Can you work these out from the model? Positions are in its coordinate system, mm. Face numbers are marked on the shaded views. A direction names the side the tool comes from. Give positions to 0.01 mm unless a question says otherwise; leave off trailing zeros. Write each loop counter-clockwise with the first axis right and the second up, starting at its lowest first coordinate (ties: lowest second). Pieces come first, ordered by that corner, then holes. Notation, with made-up numbers: M 13.5,62.25 L 25.5,62.25 A18 ccw 25.5,74.25 Z; hole C 38,-21 d7. An arc over 180 degrees is marked long. Answer as CSV lines item,"result". Start each with the question number.
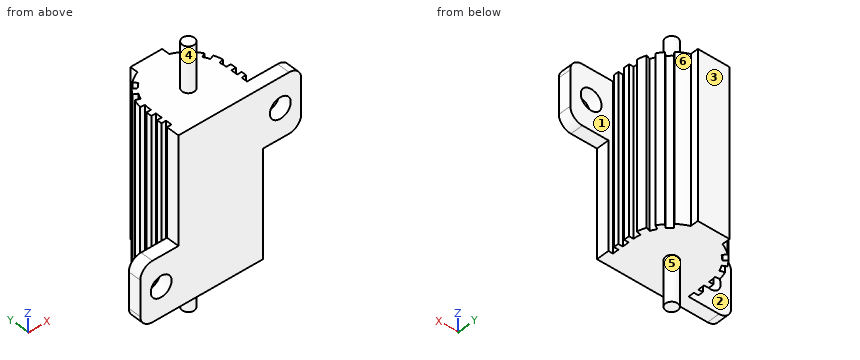
```python
from build123d import *

# Parameters (mm, degrees)
EXTRUDE1_DEPTH     = 14
SKETCH4_W          = 6.4
SKETCH4_H          = 10
EXTRUDE8_DEPTH     = 2.159
FILLET1_R          = 2.032
CUT_EXTRUDE1_START = -28
SKETCH3_W          = 0.762
SKETCH3_H          = 1.095986398
SKETCH3_H_2        = 1.017694432
CUT_EXTRUDE1_DEPTH = 28
SKETCH5_R          = 1.75
CUT_EXTRUDE2_DEPTH = 3.159
SKETCH6_R          = 1.02616
EXTRUDE9_DEPTH     = 7.62


with BuildPart() as part:
    # Sketch2 → Extrude1 (new body, symmetric)
    with BuildSketch(Plane.XY):
        with BuildLine():
            Line((-7.1, 0), (7.1, 0))
            Line((7.1, 0), (7.1, 6.096))
            ThreePointArc((7.1, 6.096), (5.887891848, 10.063710875), (2.665428286, 12.676690849))
            Line((2.665428286, 12.676690849), (2.665428286, 14))
            Line((2.665428286, 14), (-2.665428286, 14))
            Line((-2.665428286, 14), (-2.665428286, 12.676690849))
            ThreePointArc((-2.665428286, 12.676690849), (-5.887891848, 10.063710875), (-7.1, 6.096))
            Line((-7.1, 6.096), (-7.1, 0))
        make_face()
    extrude(amount=EXTRUDE1_DEPTH, both=True)

    # Sketch4 → Extrude8 (add)
    with BuildSketch(Plane.XZ):
        with Locations((-10.3, -9)):
            Rectangle(SKETCH4_W, SKETCH4_H)
        with Locations((10.3, 9)):
            Rectangle(SKETCH4_W, SKETCH4_H)
    extrude(amount=-EXTRUDE8_DEPTH)

    # Fillet1
    fillet1_edges = [part.edges().sort_by_distance(p)[0] for p in [
        (-13.5, 1.0795, -14),
        (-13.5, 1.0795, -4),
        (13.5, 1.0795, 14),
        (13.5, 1.0795, 4),
    ]]
    fillet(fillet1_edges, radius=FILLET1_R)

    # Sketch3 → Cut-Extrude1 (cut)
    with BuildSketch(Plane.XY.offset(14).offset(CUT_EXTRUDE1_START)):
        with Locations((6.719, 4.552283628)):
            Rectangle(SKETCH3_W, SKETCH3_H)
        with BuildLine():
            Line((6.236968685, 7.223149334), (6.986821973, 7.358663344))
            ThreePointArc((6.986821973, 7.358663344), (7.071648889, 6.729862758), (7.1, 6.096))
            Line((7.1, 6.096), (7.1, 6.032119719))
            Line((7.1, 6.032119719), (6.338, 6.032119719))
            Line((6.338, 6.032119719), (6.338, 6.096))
            ThreePointArc((6.338, 6.096), (6.312691642, 6.661834107), (6.236968685, 7.223149334))
        make_face()
        with Locations((6.719, 2.667847216)):
            Rectangle(SKETCH3_W, SKETCH3_H_2)
        with BuildLine():
            Line((4.012570752, 11.002069706), (4.462775162, 11.618104477))
            ThreePointArc((4.462775162, 11.618104477), (4.915642764, 11.219129534), (5.332989208, 10.783134104))
            Line((5.332989208, 10.783134104), (4.752139233, 10.289735412))
            ThreePointArc((4.752139233, 10.289735412), (4.396804558, 10.660904564), (4.012570752, 11.002069706))
        make_face()
        with BuildLine():
            Line((5.381940738, 9.443380752), (6.039888527, 9.828257571))
            ThreePointArc((6.039888527, 9.828257571), (6.330841034, 9.310102022), (6.577443928, 8.769430636))
            Line((6.577443928, 8.769430636), (5.85354185, 8.526286364))
            ThreePointArc((5.85354185, 8.526286364), (5.636424644, 8.994441172), (5.381940738, 9.443380752))
        make_face()
    cut_extrude1 = extrude(amount=CUT_EXTRUDE1_DEPTH, mode=Mode.SUBTRACT)

    # Mirror2: Cut-Extrude1 across plane
    add(cut_extrude1.mirror(Plane(origin=(0, 0, 0), x_dir=(0, 0, 1), z_dir=(1, 0, 0))), mode=Mode.SUBTRACT)

    # Sketch5 → Cut-Extrude2 (cut, through all)
    with BuildSketch(Plane(origin=(0, 2.159, 0), x_dir=(-1, 0, 0), z_dir=(0, 1, 0))):
        with Locations((-10, 9)):
            Circle(SKETCH5_R)
        with Locations((10, -9)):
            Circle(SKETCH5_R)
    extrude(amount=-CUT_EXTRUDE2_DEPTH, mode=Mode.SUBTRACT)

    # Sketch6 → Extrude9 (add)
    with BuildSketch(Plane.XY.offset(14)):
        with Locations((0, 6.096)):
            Circle(SKETCH6_R)
    extrude9 = extrude(amount=EXTRUDE9_DEPTH)

    # Mirror3: Extrude9 across plane
    add(extrude9.mirror(Plane.XY))


solid = part.part
```
1) I want a section at C-C, the plane z = -14.5. Please give me the cut outline in (x, y).
2) I'm going to push flat-ended pins straight in: P1, Ø0.9, axis at y = 4.5, z = -2, coming from the +X side; P2, Ø1.5, axis at x = 8.5, z = 16, coming from the -Y side; P3, Ø3, axis at x = -1, y = 8.5, coming from the +Z side; P4, Ø2.5, axis at x = -10, y = 1, coming from the +Z side. Where does each tip first touch, or does it pass through?
3) Thinking about a two-plate mould opening in Y: for the marked faces 1, 2, 3 and 4, which applies, released by +Y, released by -Y, zero draft, split by the parting line, or undercut?
4) I want a section at D-D, the plane x = -7.75. Please give me the cut outline in (y, z).
5) I want a section at B-B, the plane x = 0. Please give me the cut outline in (y, z).
6) I want a section at A-A, the plane x = 10. Please give me the cut outline in (y, z), then the cut area to 3 significant figures.
7) I need wall thicknesses on L1, parallel to Z at x = -10, y = 0.8; L2, parallel to Z at x = -2, y = 4.5; L3, parallel to Y at x = -6.5, z = -1.5. Which ranges of each line are inside material? Lowest first, please. Write a range as from..to.
8) On a 3-axis mill with a long thin cutter (end or side, diameter ignored), from which of +Z, -Z, +X, -X, +Y, -Y can I reach the whole of each face in a straight line? I mean the marked faces 5 and 6. Say none if no direction works.
Values found:
1,outline,"C 0,6.1 d2.05"
2,P1,"stops at x = 6.34"
2,P2,"passes through"
2,P3,"stops at z = 14"
2,P4,"stops at z = -4"
3,face 1,"undercut"
3,face 2,"undercut"
3,face 3,"released by +Y"
3,face 4,"split by the parting line"
4,outline,"M 0,-14 L 2.16,-14 L 2.16,-4 L 0,-4 Z"
5,outline,"M 0,-14 L 5.07,-14 L 5.07,-21.62 L 7.12,-21.62 L 7.12,-14 L 14,-14 L 14,14 L 7.12,14 L 7.12,21.62 L 5.07,21.62 L 5.07,14 L 0,14 Z"
6,outline,"M 0,4 L 2.16,4 L 2.16,7.25 L 0,7.25 Z; M 0,10.75 L 2.16,10.75 L 2.16,14 L 0,14 Z"
6,area,"14.0 mm²"
7,L1,"z = -14..-10.75, -7.25..-4"
7,L2,"z = -14..14"
7,L3,"y = 0..2.16, 3.18..4, 5.1..6.03, 7.27..8.74"
8,face 5,"-Z"
8,face 6,"+Z, -Z, +X, +Y"
